The drawing under review shows one solid part. Ordinate dimensions are in mm from its lowest x, y, z. A direction names the side the tool comes from. Round coordinates to 2 decimals unless told otherwise and drop trailing zeros. Order: outer loops, then holes, each group sorted by start corner. A loop starts at its lowest first (then second) coordinate and runs counter-clockwise, first axis right, second up.
1) To check wall thickness, follow L1, parallel to X at y = 10.25, z = 57.15; L2, parallel to Z at x = 57.15, y = 13.75; L3, parallel to Y at x = 47, z = 90. State the ranges of each line that lie inside material, in increasing order.
2) Clearance check with flat-ended pins moving along their axes: P1, Ø5, axis at y = 68, z = 69, coming from the -X side (1 decimal); P2, Ø5, axis at x = 90.5, z = 101, coming from the +Y side; P3, Ø6, axis at y = 83, z = 50, coming from the -X side. State where each tip first meets the part, or that it passes through.
3) Consider section B-B (x = 97.5). Give the boundary of the cut face in (y, z).
4) Consider section C-C (y = 101). Give the boundary of the cut face in (x, z).
5) Machinability: for the marked faces 1 and 2, which of the approach directions +Z, -Z, +X, -X, +Y, -Y give a long, thin tool a straight path to every point of the face, cutting with its end or side? Answer none if there is none.
6) Consider section D-D (z = 73.5). Give the boundary of the cut face in (x, y).
7) Consider section A-A (y = 10). Give the boundary of the cut face in (x, z), then the cut area to 3 significant figures.
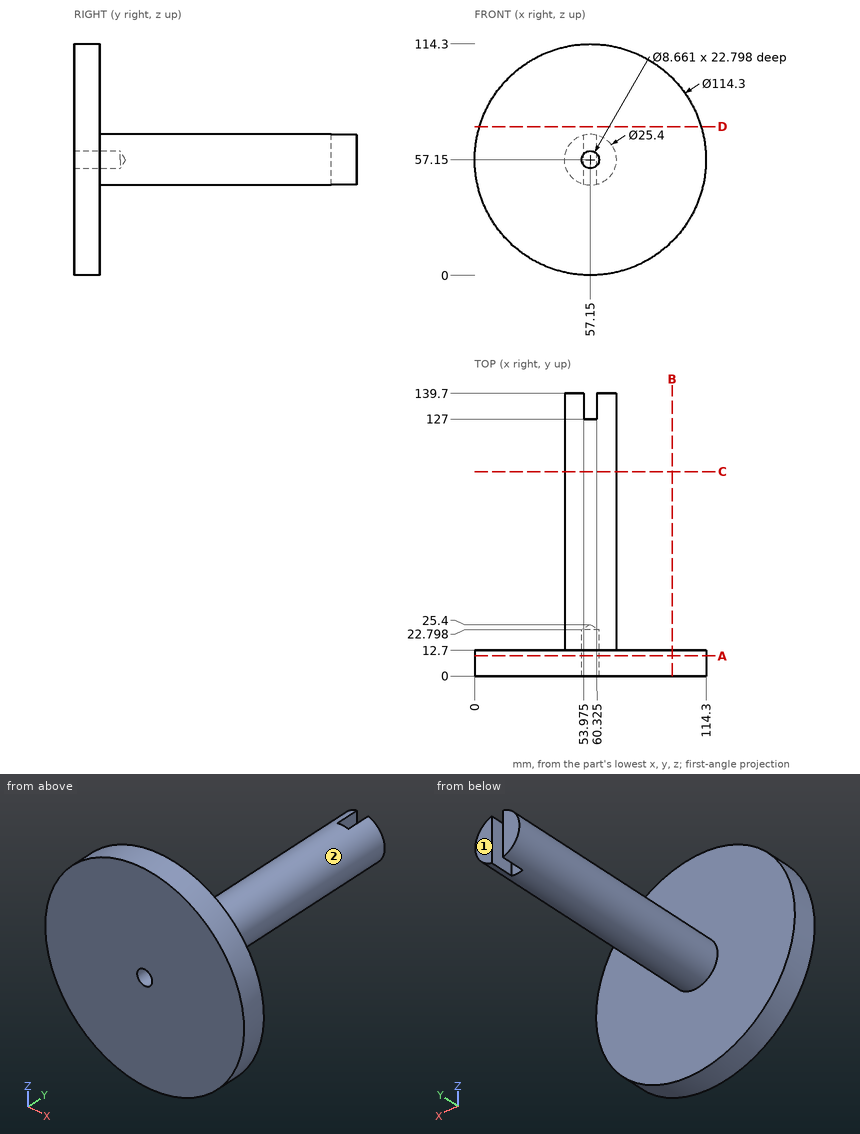
Answer below:
1. L1: x = 0 to 52.82, 61.48 to 114.3
1. L2: z = 44.45 to 52.82, 61.48 to 69.85
1. L3: y = 0 to 12.7
2. P1: stops at x = 48.6
2. P2: stops at y = 12.7
2. P3: stops at x = 45.15
3. outline: (0, 16.68) - (12.7, 16.68) - (12.7, 97.62) - (0, 97.62) - close
4. outline: circle Ø25.4 at (57.15, 57.15)
5. face 1: +Z, -Z, +X, -X, +Y
5. face 2: +Y
6. outline: (2.39, 0) - (111.91, 0) - (111.91, 12.7) - (2.39, 12.7) - close
7. outline: circle Ø114.3 at (57.15, 57.15); hole circle Ø8.66 at (57.15, 57.15)
7. area: 10,200 mm2
